Verification items for the finished model (mm, model axes). A direction names the side the tool comes from. Coordinates: 2 decimals unless noted, no trailing zeros. Order: outer loops, then holes, each group sorted by start corner. A loop starts at its lowest first (then second) coordinate and runs counter-clockwise, first axis right, second up. Notation, with made-up numbers: (66, 77.5) -> (110, 77.5) arc R10 ccw to (110, 94.5) -> close; hole circle Ø5 at (46.25, 13.5). An arc over 180 degrees is marked (long way). Write item = value, one per line. Start each with the question number.
1. Cross-section at C-C on y = 4.25. Record the cut outline in (x, z).
2. Release check for a two-part mould opening along X. For faces 1 (the flat face through (13, 44.75, 1)), 2 (the flat face through (15, 3, 1)), 3 (the cylindrical face through (-11.91, 51.99, 1.48)), 4 (the cylindrical face through (-12.74, 3.49, 1.48)) record: +X half, -X half, draft (parallel to the pull), parting line (faces both ways), or undercut.
3. Cross-section at A-A on y = 50.75. Record the cut outline in (x, z).
4. Thickness scan on line 1 along Y through (x, z) = (-11.75, 1.9); line 2 along X through (y, z) = (53, 8); line 3 along Y through (x, z) = (-12.5, 0.75). Record the ranges inside material, lowest first. Write a range as from..to.
5. Go/stop test with flat-tipped pins: P1, Ø1, axis at x = 2, z = 9, coming from the -Y side; P2, Ø3.5, axis at x = 13.5, z = 1.5, coming from the +Y side; P3, Ø0.5, axis at x = 4, y = 55.5, coming from the -Z side. Record where each tip stops, or that it passes through.
6. Cross-section at D-D on y = 26. Record the cut outline in (x, z), plus the area to 3 significant figures.
7. Set-up check for faces 5 (the flat face through (13, 6.75, 1)), 6 (the flat face through (0, 55, 3)), 7 (the flat face through (7.5, 52, 9)), 8 (the flat face through (-3.9, 55.5, 9.45)), 9 (the flat face through (0, 48, 10)): record each of +Z, -Z, +X, -X, +Y, -Y from which the full face is reachable in a straight line by a thin tool's end or side.
8. Cross-section at B-B on z = 8. Record the cut outline in (x, y).
from build123d import *

# Parameters (mm, degrees)
SKETCH1_R              = 1.25
MAIN_DEPTH             = 3
MAKERBEAMSUPPORT_DEPTH = 7.5
FILLET1_R              = 3
FILLET2_R              = 2
SKETCH3_R              = 1.5
CUT_EXTRUDE1_DEPTH     = 57


with BuildPart() as part:
    # Sketch1 → Main (new body)
    with BuildSketch(Plane.XY):
        Polygon((-15, 55), (-15, 44.75), (-11.25, 44.75), (-11.25, 6.75), (-15, 6.75), (-15, 0), (15, 0), (15, 6.75), (11.25, 6.75), (11.25, 44.75), (15, 44.75), (15, 55), align=None)
        with Locations((-11.75, 50.75)):
            Circle(SKETCH1_R, mode=Mode.SUBTRACT)
        with Locations((11.75, 50.75)):
            Circle(SKETCH1_R, mode=Mode.SUBTRACT)
        with Locations((11.75, 4.25)):
            Circle(SKETCH1_R, mode=Mode.SUBTRACT)
        with Locations((-11.75, 4.25)):
            Circle(SKETCH1_R, mode=Mode.SUBTRACT)
    extrude(amount=MAIN_DEPTH)

    # Sketch2 → MakerBeamSupport (add, symmetric)
    with BuildSketch(Plane(origin=(0, 0, 0), x_dir=(0, 0, -1), z_dir=(1, 0, 0))):
        Polygon((-13, 55), (-9.45, 55), (-9.45, 56), (-6.55, 56), (-6.55, 55), (-3, 55), (-3, 48), (-13, 48), align=None)
    extrude(amount=MAKERBEAMSUPPORT_DEPTH, both=True)

    # Fillet1
    fillet1_edges = [part.edges().sort_by_distance(p)[0] for p in [
        (0, 48, 3),
    ]]
    fillet(fillet1_edges, radius=FILLET1_R)

    # Fillet2
    fillet2_edges = [part.edges().sort_by_distance(p)[0] for p in [
        (-7.5, 51.5, 3),
        (7.5, 51.5, 3),
    ]]
    fillet(fillet2_edges, radius=FILLET2_R)

    # Sketch3 → Cut-Extrude1 (cut, through all)
    with BuildSketch(Plane(origin=(0, 56, 0), x_dir=(1, 0, 0), z_dir=(0, 1, 0))):
        with Locations((0, -8)):
            Circle(SKETCH3_R)
    extrude(amount=-CUT_EXTRUDE1_DEPTH, mode=Mode.SUBTRACT)


solid = part.part
Worked out:
q1.outline = (-15, 0) -> (-13, 0) -> (-13, 3) -> (-15, 3) -> close; (-10.5, 0) -> (10.5, 0) -> (10.5, 3) -> (-10.5, 3) -> close; (13, 0) -> (15, 0) -> (15, 3) -> (13, 3) -> close
q2.face_1 = draft
q2.face_2 = +X half
q2.face_3 = undercut
q2.face_4 = undercut
q3.outline = (-15, 0) -> (-13, 0) -> (-13, 3) -> (-15, 3) -> close; (-10.5, 0) -> (10.5, 0) -> (10.5, 3) -> (9.5, 3) arc R2 cw to (7.5, 5) -> (7.5, 13) -> (-7.5, 13) -> (-7.5, 5) arc R2 cw to (-9.5, 3) -> (-10.5, 3) -> close; (13, 0) -> (15, 0) -> (15, 3) -> (13, 3) -> close; hole circle Ø3 at (0, 8)
q4.line_1 = 0..3, 5.5..6.75, 44.75..49.5, 52..55
q4.line_2 = -7.5..-1.5, 1.5..7.5
q4.line_3 = 0..3.25, 5.25..6.75, 44.75..49.75, 51.75..55
q5.P1 = 48
q5.P2 = 55
q5.P3 = 6.55
q6.outline = (-11.25, 0) -> (11.25, 0) -> (11.25, 3) -> (-11.25, 3) -> close
q6.area = 67.5 mm²
q7.face_5 = +Z, -Z, +X
q7.face_6 = -Z, +X, -X, +Y
q7.face_7 = +Z, +X, +Y, -Y
q7.face_8 = +Z, +X, -X, +Y
q7.face_9 = +Z, +X, -X, -Y
q8.outline = (-7.5, 48) -> (-1.5, 48) -> (-1.5, 56) -> (-7.5, 56) -> close; (1.5, 48) -> (7.5, 48) -> (7.5, 56) -> (1.5, 56) -> close
